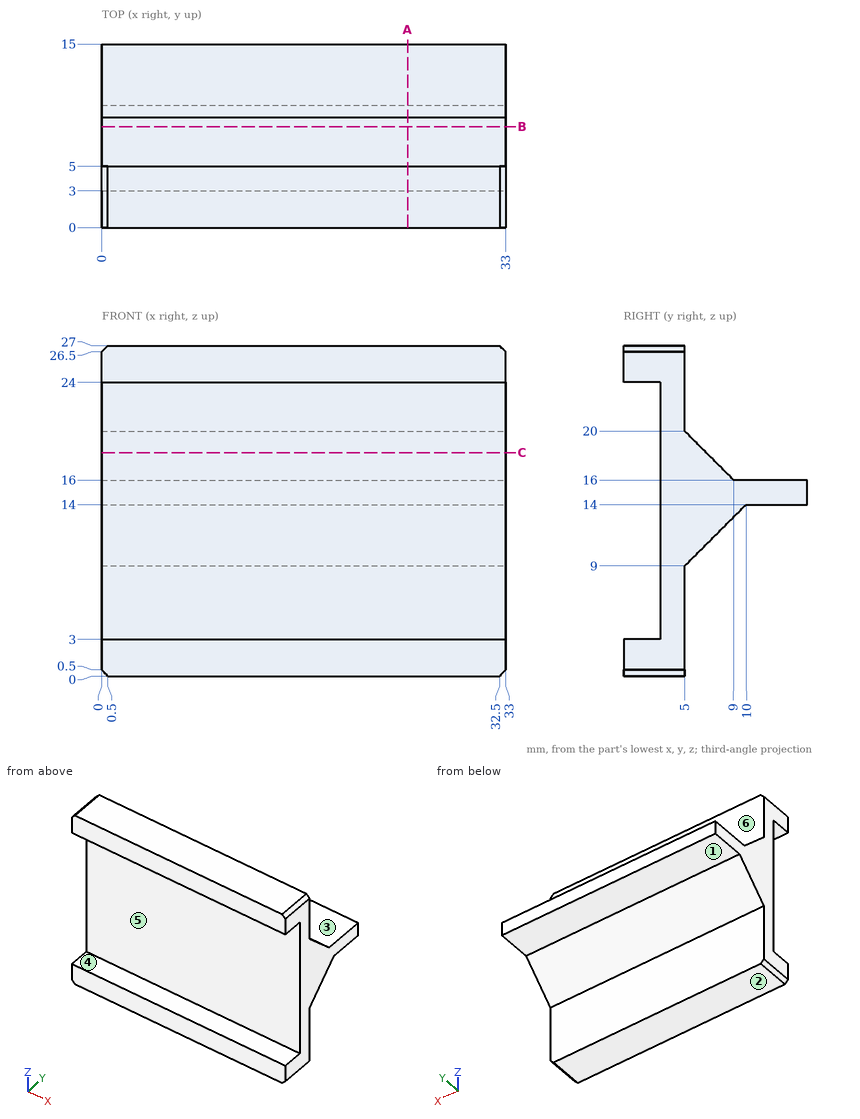
Source: three-view drawing plus pictorial views. Frame: mm from the lowest corner of the part. A direction names the side the tool comes from. Round coordinates to 2 decimals unless told otherwise and drop trailing zeros. Order: outer loops, then holes, each group sorted by start corner. A loop starts at its lowest first (then second) coordinate and runs counter-clockwise, first axis right, second up. Notation, with made-up numbers: (50, 1) -> (71, 1) arc R16 ccw to (71, 7) -> close; hole circle Ø2 at (56.25, 40). An arc over 180 degrees is marked (long way). Use one line per item in the form item = value. Start each with the question number.
1. Cut plane B-B (y = 8.25). Return the cut outline in (x, z), then the cut area to 4 significant figures.
2. Draft query along Z for the marked faces 3, 4, 5 and 6. Return one class per face: pulls with the +Z half, pulls with the -Z half, needs draft (parallel to the pull), parting line crosses it, or undercut.
3. Reachability of the marked faces 1 and 2 from +Z, -Z, +X, -X, +Y, -Y: full face, straight path, thin tool, end or side. Return the list, or none.
4. Cut plane C-C (z = 18.25). Return the cut outline in (x, y), then the cut area to 3 significant figures.
5. Pin query (flat end, axial travel): pin 1 Ø2.5 at (x, y) = (9, 11.5) entering from -Z; pin 2 Ø7.5 at (x, z) = (16.5, 24.5) entering from +Y; pin 3 Ø1 at (x, y) = (22, 8) entering from -Z; pin 4 Ø6 at (y, z) = (12, 16.5) entering from +X. Return the tip coordinate at first contact, or that it passes through.
6. Cut plane A-A (x = 25). Return the cut outline in (y, z), then the cut area to 4 significant figures.
7. Line query: probe 1 along Z at (x, y) = (31, 2.5); probe 2 along Y at (x, z) = (6, 23); probe 3 along Y at (x, z) = (5, 15.25). Output: solid intervals per line, ascending.
Solution:
q1.outline = (0, 12.25) -> (33, 12.25) -> (33, 16.75) -> (0, 16.75) -> close
q1.area = 148.5 mm^2
q2.face_3 = pulls with the +Z half
q2.face_4 = undercut
q2.face_5 = undercut
q2.face_6 = needs draft
q3.face_1 = -Z, +X, -X, +Y
q3.face_2 = -Z, +X, -X, +Y, -Y
q4.outline = (0, 3) -> (33, 3) -> (33, 6.75) -> (0, 6.75) -> close
q4.area = 124 mm^2
q5.pin_1 = 14
q5.pin_2 = 5
q5.pin_3 = 11.5
q5.pin_4 = 33
q6.outline = (0, 0) -> (5, 0) -> (5, 9) -> (10, 14) -> (15, 14) -> (15, 16) -> (9, 16) -> (5, 20) -> (5, 27) -> (0, 27) -> (0, 24) -> (3, 24) -> (3, 3) -> (0, 3) -> close
q6.area = 112.5 mm^2
q7.probe_1 = 0 to 3, 24 to 27
q7.probe_2 = 3 to 5
q7.probe_3 = 3 to 15
